from build123d import *

# Parameters (mm, degrees)
SKETCH1_2_R                 = 1.6383
BOSS_EXTRUDE2_DEPTH         = 1.575
SKETCH2_W                   = 14.080651801
SKETCH2_H                   = 7.11628052
SKETCH2_W_2                 = 15.007196354
SKETCH2_H_2                 = 9.421332762
CUT_EXTRUDE1_DEPTH          = 65.400942629
ADDITIONAL_PCB_MATERIAL_W   = 2.649520344
ADDITIONAL_PCB_MATERIAL_H   = 65.213315835
ADDITIONAL_PCB_MATERIAL_W_2 = 1.5
ADDITIONAL_PCB_MATERIAL_H_2 = 65.299191064
BOSS_EXTRUDE3_DEPTH         = 1.575
SKETCH3_W                   = 46.818
SKETCH3_H                   = 1
BOSS_EXTRUDE4_DEPTH         = 1.575
SKETCH4_W                   = 2
SKETCH4_H                   = 2.5
CUT_EXTRUDE2_DEPTH          = 65.400942629
SKETCH5_W                   = 2.5
SKETCH5_H                   = 18.09999695
SKETCH5_H_2                 = 19.499999394
BOSS_EXTRUDE5_DEPTH         = 1.575
SKETCH7_W                   = 9.5
SKETCH7_H                   = 1.20600305
CUT_EXTRUDE3_DEPTH          = 65.400942629
M3_CLEARANCE_HOLE1_D        = 3.2
M3_CLEARANCE_HOLE2_D        = 3.2
M3_CLEARANCE_HOLE3_D        = 3.2
M3_CLEARANCE_HOLE4_D        = 3.2
M3_CLEARANCE_HOLE5_D        = 3.2
SKETCH26_W                  = 2.575
SKETCH26_H                  = 5
CUT_EXTRUDE4_DEPTH          = 10


with BuildPart() as part:
    # Sketch1_2 → Boss-Extrude2 (new body)
    with BuildSketch(Plane(origin=(0, 0, 0), x_dir=(1, 0, 0), z_dir=(0, 1, 0))):
        with BuildLine():
            Line((-38.39500299, 29.999999735), (-42.73000299, 29.999999735))
            Line((-42.73000299, 29.999999735), (-43.011025994, 30.003097626))
            ThreePointArc((-43.011025994, 30.003097626), (-43.710996344, 30.299838092), (-44.000003042, 31.003036872))
            Line((-44.000003042, 31.003036872), (-44.000003042, 31.269999735))
            Line((-44.000003042, 31.269999735), (-44.000005679, 44.999999735))
            ThreePointArc((-44.000005679, 44.999999735), (-43.414218633, 46.414215608), (-42.000002924, 47.000003051))
            Line((-42.000002924, 47.000003051), (-30.435003, 47.000003051))
            Line((-30.435003, 47.000003051), (-30.435003, 22.255357341))
            Line((-30.435003, 22.255357341), (-11.409003, 22.255357341))
            Line((-11.409003, 22.255357341), (-11.409003, -9.899999999))
            Line((-11.409003, -9.899999999), (-23.409003, -9.899999999))
            Line((-23.409003, -9.899999999), (-23.409003, -31.499996949))
            Line((-23.409003, -31.499996949), (23.408997, -31.499996949))
            Line((23.408997, -31.499996949), (23.408997, -8.499997555))
            Line((23.408997, -8.499997555), (11.97084713, -8.499997555))
            Line((11.97084713, -8.499997555), (11.97084713, 22.255357341))
            Line((11.97084713, 22.255357341), (30.434997, 22.255357341))
            Line((30.434997, 22.255357341), (30.434997, 47.000003051))
            Line((30.434997, 47.000003051), (42.000008541, 47.000003051))
            ThreePointArc((42.000008541, 47.000003051), (43.414213215, 46.414220704), (43.999996956, 45.000016607))
            Line((43.999996956, 45.000016607), (43.999996956, 32.000003378))
            Line((43.999996956, 32.000003378), (43.999996956, 31.015615364))
            ThreePointArc((43.999996956, 31.015615364), (43.706534093, 30.307939396), (42.998386406, 30.015616661))
            Line((42.998386406, 30.015616661), (33.825607551, 30.030389905))
            ThreePointArc((33.825607551, 30.030389905), (33.117459864, 29.738067169), (32.823997, 29.030391202))
            Line((32.823997, 29.030391202), (32.823997, -30.453996949))
            ThreePointArc((32.823997, -30.453996949), (33.116890219, -31.16110373), (33.823997, -31.453996949))
            Line((33.823997, -31.453996949), (36.099999555, -31.453996949))
            Line((36.099999555, -31.453996949), (42.849728118, -31.453996949))
            ThreePointArc((42.849728118, -31.453996949), (43.556834899, -31.746890168), (43.849728118, -32.453996949))
            Line((43.849728118, -32.453996949), (43.849728118, -36.999996949))
            Line((43.849728118, -36.999996949), (43.849728118, -46.999996949))
            Line((43.849728118, -46.999996949), (-42.000000178, -46.999996949))
            ThreePointArc((-42.000000178, -46.999996949), (-43.414212804, -46.414211581), (-44.000000499, -44.999999921))
            Line((-44.000000499, -44.999999921), (-44.000000178, -38.976999921))
            Line((-44.000000178, -38.976999921), (-44.000000178, -32.453999802))
            ThreePointArc((-44.000000178, -32.453999802), (-43.70710696, -31.746893021), (-43.000000178, -31.453999802))
            Line((-43.000000178, -31.453999802), (-36.100000549, -31.453999802))
            Line((-36.100000549, -31.453999802), (-33.824003042, -31.453999802))
            ThreePointArc((-33.824003042, -31.453999802), (-33.116896261, -31.161106583), (-32.824003042, -30.453999802))
            Line((-32.824003042, -30.453999802), (-32.824003042, 29.011483943))
            ThreePointArc((-32.824003042, 29.011483943), (-33.117785331, 29.719478678), (-33.826516131, 30.011480785))
            Line((-33.826516131, 30.011480785), (-38.39500299, 29.999999735))
        make_face()
        with Locations(Location((40, 43.5, 0), (0, 0, 270))):
            Circle(SKETCH1_2_R, mode=Mode.SUBTRACT)
        with Locations(Location((-40, 43.5, 0), (0, 0, 270))):
            Circle(SKETCH1_2_R, mode=Mode.SUBTRACT)
        with Locations(Location((-37.6, -42.2, 0), (0, 0, 270))):
            Circle(SKETCH1_2_R, mode=Mode.SUBTRACT)
        with Locations(Location((36.1, -42.2, 0), (0, 0, 270))):
            Circle(SKETCH1_2_R, mode=Mode.SUBTRACT)
    extrude(amount=BOSS_EXTRUDE2_DEPTH)

    # Sketch2 → Cut-Extrude1 (cut, through all)
    with BuildSketch(Plane(origin=(0, 1.575, 0), x_dir=(1, 0, 0), z_dir=(0, 1, 0))):
        with Locations((39.863054019, -29.135856689)):
            Rectangle(SKETCH2_W, SKETCH2_H)
        with Locations((-40.336598676, -27.983330568)):
            Rectangle(SKETCH2_W_2, SKETCH2_H_2)
    extrude(amount=-CUT_EXTRUDE1_DEPTH, mode=Mode.SUBTRACT)

    # Additional PCB material → Boss-Extrude3 (add)
    with BuildSketch(Plane(origin=(0, 1.575, 0), x_dir=(1, 0, 0), z_dir=(0, 1, 0))):
        with Locations((32.999236828, -1.128517583)):
            Rectangle(ADDITIONAL_PCB_MATERIAL_W, ADDITIONAL_PCB_MATERIAL_H)
        with Locations((-33.574003042, -1.085579968)):
            Rectangle(ADDITIONAL_PCB_MATERIAL_W_2, ADDITIONAL_PCB_MATERIAL_H_2)
    extrude(amount=-BOSS_EXTRUDE3_DEPTH)

    # Sketch3 → Boss-Extrude4 (add)
    with BuildSketch(Plane(origin=(0, 1.575, 0), x_dir=(1, 0, 0), z_dir=(0, 1, 0))):
        with Locations((-3e-06, -30.999996949)):
            Rectangle(SKETCH3_W, SKETCH3_H)
    extrude(amount=-BOSS_EXTRUDE4_DEPTH)

    # Sketch4 → Cut-Extrude2 (cut, through all)
    with BuildSketch(Plane(origin=(0, 1.575, 0), x_dir=(1, 0, 0), z_dir=(0, 1, 0))):
        with Locations((24.408997, -29.249996949)):
            Rectangle(SKETCH4_W, SKETCH4_H)
        with Locations((-24.409003, -29.249996949)):
            Rectangle(SKETCH4_W, SKETCH4_H)
    extrude(amount=-CUT_EXTRUDE2_DEPTH, mode=Mode.SUBTRACT)

    # Sketch5 → Boss-Extrude5 (add)
    with BuildSketch(Plane(origin=(0, 1.575, 0), x_dir=(1, 0, 0), z_dir=(0, 1, 0))):
        with Locations((-22.159003, -18.949998474)):
            Rectangle(SKETCH5_W, SKETCH5_H)
        with Locations((22.158997, -18.249997252)):
            Rectangle(SKETCH5_W, SKETCH5_H_2)
    extrude(amount=-BOSS_EXTRUDE5_DEPTH)

    # Sketch7 → Cut-Extrude3 (cut, through all)
    with BuildSketch(Plane(origin=(0, 1.575, 0), x_dir=(1, 0, 0), z_dir=(0, 1, 0))):
        with Locations((-16.159003, -9.296998474)):
            Rectangle(SKETCH7_W, SKETCH7_H)
    extrude(amount=-CUT_EXTRUDE3_DEPTH, mode=Mode.SUBTRACT)

    # M3 Clearance Hole1 (through all)
    with Locations(Plane(origin=(-37.357724691, 1.575, 48.235847646), x_dir=(-1, 0, 0), z_dir=(0, 1, 0))):
        with Locations((-23.558721691, -42.724316051), (-23.558721691, -67.244316051), (-7.038721691, -67.244316051), (-7.038721691, -42.724316051)):
            Hole(M3_CLEARANCE_HOLE1_D / 2)

    # M3 Clearance Hole2 (through all)
    with Locations(Plane(origin=(-37.357724691, 1.575, 48.235847646), x_dir=(-1, 0, 0), z_dir=(0, 1, 0))):
        with Locations((-51.71857182, -42.724316051)):
            Hole(M3_CLEARANCE_HOLE2_D / 2)

    # M3 Clearance Hole3 (through all)
    with Locations(Plane(origin=(-37.357724691, 1.575, 48.235847646), x_dir=(-1, 0, 0), z_dir=(0, 1, 0))):
        with Locations((-68.23857182, -42.724316051)):
            Hole(M3_CLEARANCE_HOLE3_D / 2)

    # M3 Clearance Hole4 (through all)
    with Locations(Plane(origin=(-37.357724691, 21.15, 48.235847646), x_dir=(-1, 0, 0), z_dir=(0, 1, 0))):
        with Locations((-51.71857182, -67.244316051)):
            Hole(M3_CLEARANCE_HOLE4_D / 2)

    # M3 Clearance Hole5 (through all)
    with Locations(Plane(origin=(-37.357724691, 1.575, 48.235847646), x_dir=(-1, 0, 0), z_dir=(0, 1, 0))):
        with Locations((-68.23857182, -67.244316051)):
            Hole(M3_CLEARANCE_HOLE5_D / 2)

    # Sketch26 → Cut-Extrude4 (cut)
    with BuildSketch(Plane(origin=(0, 1.575, 0), x_dir=(1, 0, 0), z_dir=(0, 1, 0))):
        Polygon((-36.984003042, 35.010230552), (-34.324003042, 35.010230552), (-34.324003042, 29.927765717), (-36.984003042, 29.927765717), (-36.984003042, 30.010230552), align=None)
        with Locations((35.612496956, 32.515616661)):
            Rectangle(SKETCH26_W, SKETCH26_H)
    extrude(amount=-CUT_EXTRUDE4_DEPTH, mode=Mode.SUBTRACT)


solid = part.part
CAD build for the part. Positions are in the model's coordinates, mm. Coordinates: 2 decimals unless noted, no trailing zeros. Write each loop counter-clockwise with the first axis right and the second up, starting at its lowest first coordinate (ties: lowest second). Pieces come first, ordered by that corner, then holes. Notation, with made-up numbers: M 59.5,25.25 L 102.5,25.25 A17 cw 102.5,46.25 Z; hole C 9,13.25 d5. An arc over 180 degrees is marked long. Return JSON: item names as keys, results as strings.
Item 1: Slice it at D-D, the plane z = -11. Write the cut outline in (x, y) (3 decimals).
Findings below:
{"outline": "M -34.324,0 L -11.409,0 L -11.409,1.575 L -34.324,1.575 Z; M 11.971,0 L 34.324,0 L 34.324,1.575 L 11.971,1.575 Z"}
Item 2: Drop flat-ended pins along their axis: pin 1 Ø0.5 at (x, y) = (7.5, 1) entering from -Z; pin 2 Ø0.8 at (y, z) = (0.5, -4) entering from +X; pin 3 Ø4 at (x, z) = (-37.6, 42.2) entering from -Y; pin 4 Ø2.5 at (x, z) = (-40, -43.5) entering from +Y. Give the stop position or say it passes through.
Findings below:
{"pin 1": "stops at z = 30.5", "pin 2": "stops at x = 34.32", "pin 3": "stops at y = 0", "pin 4": "passes through"}
Item 3: Slice it at A-A, the plane z = 42.2. Write the cut outline in (x, y) (3 decimals), and give its area (3 significant figures).
Findings below:
{"outline": "M -44,0 L -39.238,0 L -39.238,1.575 L -44,1.575 Z; M -35.962,0 L 34.462,0 L 34.462,1.575 L -35.962,1.575 Z; M 37.738,0 L 43.85,0 L 43.85,1.575 L 37.738,1.575 Z", "area": "128 mm2"}
Item 4: Probe line 1 (X direction, y = 1.3, z = -32.5) (3 decimals); line 2 (X direction, y = 1, z = 42.2); line 3 (Z direction, x = 16.5, y = 1.15). List the from-to ranges inside material, lowest first. Write a range as from..to.
Findings below:
{"line 1": "x = -44..-36.984, -34.324..-30.435, 30.435..34.325, 36.9..44", "line 2": "x = -44..-39.24, -35.96..34.46, 37.74..43.85", "line 3": "z = -22.26..8.5, 30.5..47"}
Item 5: Slice it at C-C, the plane z = -43.5. Write the cut outline in (x, y) (3 decimals), and give its area (3 significant figures).
Findings below:
{"outline": "M -44,0 L -41.638,0 L -41.638,1.575 L -44,1.575 Z; M -38.362,0 L -30.435,0 L -30.435,1.575 L -38.362,1.575 Z; M 30.435,0 L 38.362,0 L 38.362,1.575 L 30.435,1.575 Z; M 41.638,0 L 44,0 L 44,1.575 L 41.638,1.575 Z", "area": "32.4 mm2"}
Item 6: Slice it at B-B, the plane x = 18. Write the cut outline in (y, z) (3 decimals).
Findings below:
{"outline": "M 0,-22.255 L 1.575,-22.255 L 1.575,8.5 L 0,8.5 Z; M 0,30.5 L 1.575,30.5 L 1.575,47 L 0,47 Z"}
Item 7: Two-plate mould, pull along Z, no slides. Class faces 1 (the cylindrical face through (-43.43, 0.78, -46.4)), 2 (the cylindrical face through (-12.32, 0.78, 4.9)), 3 (the flat face through (-1, 1.575, 31)): +Z half, -Z half, draft (parallel to the pull), parting line (faces both ways), or undercut.
Findings below:
{"face 1": "-Z half", "face 2": "undercut", "face 3": "draft"}
